from build123d import *

# Parameters (mm, degrees)
F1_DEPTH = 63.5
F0_W     = 26.6352667648
F0_H     = 19.05
F2_DEPTH = 25.4
F3_DEPTH = 7.9375
F5_R     = 6.35


with BuildPart() as f1:
    # F0 (on Front) → F1 (new body, symmetric)
    with BuildSketch(Plane.XZ):
        Polygon((-41.275, 9.525), (-41.275, -9.525), (41.275, -9.525), (41.275, 9.525), (22.225, 9.525), align=None)
    extrude(amount=F1_DEPTH, both=True)

    # F0 (on Front) → F2 (join, symmetric)
    with BuildSketch(Plane.XZ):
        with BuildLine():
            Line((22.225, 9.525), (41.275, 9.525))
            Line((41.275, 9.525), (41.275, 27.0002))
            ThreePointArc((41.275, 27.0002), (45.9246798487, 38.2255201513), (57.15, 42.8752))
            Line((57.15, 42.8752), (59.0897332352, 42.8752))
            Line((59.0897332352, 42.8752), (59.0897332352, 61.9252))
            Line((59.0897332352, 61.9252), (57.15, 61.9252))
            add(Edge.make_bspline(
                [(56.5390411257, 61.9198557007), (56.7424803889, 61.9218514766), (56.9461336922, 61.9236329014), (57.15, 61.9252)],
                knots=[111.1067755669, 111.1067755669, 111.1067755669, 111.1067755669, 111.5045361635, 111.5045361635, 111.5045361635, 111.5045361635], degree=3))
            ThreePointArc((56.5390411257, 61.9198557007), (32.2392255872, 51.4789447218), (22.225, 27.0002))
            Line((22.225, 27.0002), (22.225, 9.525))
        make_face()
        with Locations((72.4073666176, 52.4002)):
            Rectangle(F0_W, F0_H)
    extrude(amount=F2_DEPTH, both=True)

    # F0 (on Front) → F3 (join, symmetric)
    with BuildSketch(Plane.XZ):
        with BuildLine():
            add(Edge.make_bspline(
                [(-41.275, 9.525), (-40.4140404528, 44.079992279), (-0.2878058759, 61.3623740581), (56.5390411257, 61.9198557007)],
                knots=[0, 0, 0, 0, 111.1067755669, 111.1067755669, 111.1067755669, 111.1067755669], degree=3))
            Line((-41.275, 9.525), (22.225, 9.525))
            Line((22.225, 9.525), (22.225, 27.0002))
            ThreePointArc((22.225, 27.0002), (32.2392255872, 51.4789447218), (56.5390411257, 61.9198557007))
        make_face()
    extrude(amount=F3_DEPTH, both=True)

    # F0 (on Front) → F4 (revolve)
    with BuildSketch(Plane.XZ):
        Polygon((85.725, 66.675), (85.725, 61.9252), (85.725, 42.8752), (85.725, 38.1), (109.8897332352, 38.1), (109.8897332352, 66.675), align=None)
    revolve(axis=Axis((85.725, 0, 52.4002), (0, 0, -1)))

    # F5
    f5_edges = [f1.edges().sort_by_distance(p)[0] for p in [
        (-41.275, -63.5, 0),
        (41.275, -63.5, 0),
        (41.275, 63.5, 0),
        (-41.275, 63.5, 0),
    ]]
    fillet(f5_edges, radius=F5_R)


solid = f1.part
Read the model definition and answer for the solid it produces. Units are mm, in the model's axes. A direction names the side the tool comes from. Give positions to 0.01 mm unless a question says otherwise; leave off trailing zeros. Write each loop counter-clockwise with the first axis right and the second up, starting at its lowest first coordinate (ties: lowest second). Pieces come first, ordered by that corner, then holes. Notation, with made-up numbers: (-2.5, -6) - (43.5, -6) arc R19 ccw to (43.5, 4) - close; hole circle Ø9 at (32.25, 46). An arc over 180 degrees is marked (long way). Return JSON: item names as keys, results as strings.
Q1. A cutting plane is placed at B-B, the plane y = 34. Determine the outline of the cut face in (x, z) (3 decimals).
Reply:
{"outline": "(-41.275, -9.525) - (41.275, -9.525) - (41.275, 9.525) - (-41.275, 9.525) - close"}
Q2. For a pull along X with two mould halves and no side action, classify faces 4 (the face through (45.8, -0.4, 38.1)), 5 (the face through (46, -25.4, 42)), 6 (the face through (-39.365, -61.689, -0.133)) as released by +X, released by -X, zero draft, split by the parting line, or undercut.
Reply:
{"face 4": "undercut", "face 5": "zero draft", "face 6": "released by -X"}
Q3. A cutting plane is placed at C-C, the plane x = 99.5. Determine the outline of the cut face in (y, z) (3 decimals).
Reply:
{"outline": "(-19.854, 38.1) - (19.854, 38.1) - (19.854, 66.675) - (-19.854, 66.675) - close"}
Q4. A cutting plane is placed at A-A, the plane z = 0.5. Determine the outline of the cut face in (x, y) (3 decimals), and give its area (3 significant figures).
Reply:
{"outline": "(-41.275, -57.15) arc R6.35 ccw to (-34.925, -63.5) - (34.925, -63.5) arc R6.35 ccw to (41.275, -57.15) - (41.275, 57.15) arc R6.35 ccw to (34.925, 63.5) - (-34.925, 63.5) arc R6.35 ccw to (-41.275, 57.15) - close", "area": "10,400 mm²"}
Q5. Given P1, Ø1, axis at x = 3, z = 34.5, coming from the -Y side; P2, Ø5, axis at y = -20.5, z = 20, coming from the -X side (3 decimals); P3, Ø4, axis at y = 10.5, z = 59, coming from the -X side; P4, Ø8, axis at x = 82.5, y = 24.5, coming from the +Z side (3 decimals), each flat-ended and moving along its own axis, determine where each tip first touches the part or whether it passes through.
Reply:
{"P1": "y = -7.94", "P2": "x = 22.225", "P3": "x = 39.27", "P4": "z = 66.675"}
Q6. For faces 1 (the face through (46, 25.4, 42)), 2 (the face through (22.225, 17, 18)), 3 (the face through (61, 0, 61.925)), determine the directions among +Z, -Z, +X, -X, +Y, -Y from which every point of the face is accessible in a straight line to the end or side of a thin tool.
Reply:
{"face 1": "+Z, +X, -X, +Y", "face 2": "+Z, -X, +Y", "face 3": "+Z, -X"}
Q7. Consider line 1 along Z through (x, y) = (39.5, -40.5) (3 decimals); line 2 along X through (y, z) = (57.5, 6.5); line 3 along Z through (x, y) = (99.5, 1) (3 decimals). Determine where each line is inside the solid, lowest interval first. Write a range as [from, to].
Reply:
{"line 1": "[-9.525, 9.525]", "line 2": "[-41.27, 41.27]", "line 3": "[38.1, 66.675]"}
